from build123d import *

# Parameters (mm, degrees)
BOX201_W     = 13
BOX201_H     = 8
BOX201_DEPTH = 5
FILLET048_R  = 1
BOX203_W     = 15.5
BOX203_H     = 9.5
BOX203_DEPTH = 1.5


with BuildPart() as fillet048:
    # Box201 → Box201 (new body)
    with BuildSketch(Plane(origin=(44, 20, 6.3), x_dir=(1, 0, 0), z_dir=(0, 0, 1))):
        with Locations((6.5, 4)):
            Rectangle(BOX201_W, BOX201_H)
    extrude(amount=BOX201_DEPTH)

    # Fillet048
    fillet048_edges = [fillet048.edges().sort_by_distance(p)[0] for p in [
        (44, 24, 11.3),
        (57, 24, 11.3),
        (50.5, 20, 11.3),
        (50.5, 28, 11.3),
    ]]
    fillet(fillet048_edges, radius=FILLET048_R)


with BuildPart() as fusion062:
    # Box203 → Box203 (new body)
    with BuildSketch(Plane(origin=(42.75, 19.25, 6.3), x_dir=(1, 0, 0), z_dir=(0, 0, 1))):
        with Locations((7.75, 4.75)):
            Rectangle(BOX203_W, BOX203_H)
    extrude(amount=BOX203_DEPTH)

    # Fusion062: union Fillet048
    add(fillet048.part)


solid = fusion062.part
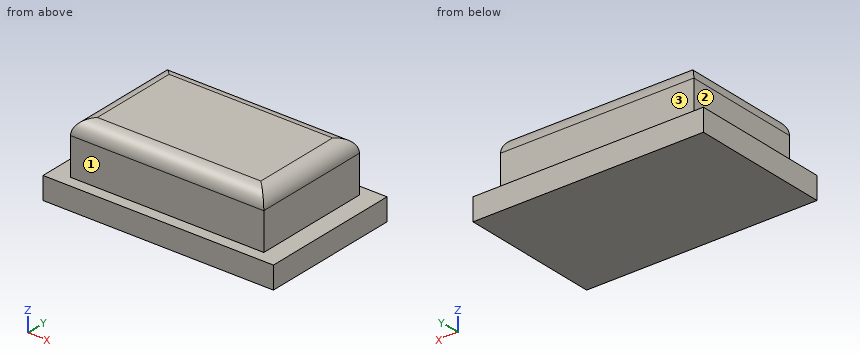
Input: part model. Units: mm. Frame: model coordinates. Face numbers are marked on the shaded views. A direction names the side the tool comes from. Coordinates: 2 decimals unless noted, no trailing zeros. Loops run counter-clockwise (first coordinate to the right, second up) from the corner with the lowest first, then second, coordinate; pieces in that order, holes last.
Q1. Material intervals for line 1 (X direction, y = 25.75, z = 8.05); line 2 (Y direction, x = 48, z = 8.8); line 3 (Z direction, x = 54, y = 19.5), sorted ascending.
Q2. Set-up query: the marked faces 1, 2 and 3. Return all of +Z, -Z, +X, -X, +Y, -Y with unobstructed straight access to the full face (end or side cutting, diameter ignored); none if empty.
Q3. Contact query for flat-ended pins moving along their axis: pin 1 (3 mm diameter, centred on x = 51.5, z = 9.5, fed in from -Y); pin 2 (1 mm diameter, centred on x = 48.5, z = 9, fed in from +Y); pin 3 (0.8 mm diameter, centred on y = 23, z = 9.5, fed in from -X). Output: stop coordinate, or through.
Q4. Cut plane C-C (z = 8.85). Output: boundary loops of the cut face in (x, y), then the cut area to 3 significant figures.
Q5. Cut plane B-B (y = 24). Output: boundary loops of the cut face in (x, z).
Q6. Cut plane D-D (x = 43.75). Output: boundary loops of the cut face in (y, z).
Q7. Cut plane A-A (x = 54.25). Output: boundary loops of the cut face in (y, z).
Working result:
1. line 1: x = 44 to 57
1. line 2: y = 20 to 28
1. line 3: z = 6.3 to 7.8
2. face 1: +Z, +X, -X, -Y
2. face 2: +Z, -X, +Y, -Y
2. face 3: +Z, +X, -X, +Y
3. pin 1: stops at y = 20
3. pin 2: stops at y = 28
3. pin 3: stops at x = 44
4. outline: (44, 20) - (57, 20) - (57, 28) - (44, 28) - close
4. area: 104 mm2
5. outline: (42.75, 6.3) - (58.25, 6.3) - (58.25, 7.8) - (57, 7.8) - (57, 10.3) arc R1 ccw to (56, 11.3) - (45, 11.3) arc R1 ccw to (44, 10.3) - (44, 7.8) - (42.75, 7.8) - close
6. outline: (19.25, 6.3) - (28.75, 6.3) - (28.75, 7.8) - (19.25, 7.8) - close
7. outline: (19.25, 6.3) - (28.75, 6.3) - (28.75, 7.8) - (28, 7.8) - (28, 10.3) arc R1 ccw to (27, 11.3) - (21, 11.3) arc R1 ccw to (20, 10.3) - (20, 7.8) - (19.25, 7.8) - close
